Work out the finished part from the listing and answer in its coordinate system (mm). A direction names the side the tool comes from. Round coordinates to 2 decimals unless told otherwise and drop trailing zeros. Order: outer loops, then holes, each group sorted by start corner. A loop starts at its lowest first (then second) coordinate and runs counter-clockwise, first axis right, second up.
from build123d import *

# Parameters (mm, degrees)
FACE_2_R                      = 17
BOSS_EXTRUDE5_DEPTH           = 2
BOSS_EXTRUDE6_START           = -56
BOSS_EXTRUDE6_OUTLINE_R       = 17
BOSS_EXTRUDE6_OUTLINE_R_2     = 10
BOSS_EXTRUDE6_DEPTH           = 54
DRIVER_PIN_BODY_CUT_START     = 9.886859906
DRIVER_PIN_BODY_CUT_OUTLINE_R = 1.5
DRIVER_PIN_BODY_CUT_DEPTH     = 6.113140094
SKETCH5_R                     = 10
SKETCH5_R_2                   = 5
BOSS_EXTRUDE7_DEPTH           = 2
DRIVER_PIN_SKETCH_R           = 1
DRIVER_PIN_SKETCH_R_2         = 0.15
DRIVER_PIN_NECK_EXTRUDE_DEPTH = 1
SKETCH5_6_R                   = 5
SKETCH5_6_R_2                 = 2
CUT_EXTRUDE1_DEPTH            = 1


# Read off the part's stored shape, not the designer's step: Boss-Extrude6, driver_pin_body_cut
with BuildPart() as part:
    # face 2 → Boss-Extrude5 (new body)
    with BuildSketch(Plane.XY):
        Circle(FACE_2_R)
    extrude(amount=-BOSS_EXTRUDE5_DEPTH)

    # Boss-Extrude6 outline → Boss-Extrude6 (add)
    with BuildSketch(Plane.XY.offset(BOSS_EXTRUDE6_START)):
        Circle(BOSS_EXTRUDE6_OUTLINE_R)
        Circle(BOSS_EXTRUDE6_OUTLINE_R_2, mode=Mode.SUBTRACT)
    extrude(amount=BOSS_EXTRUDE6_DEPTH)

    # driver_pin_body_cut outline → driver_pin_body_cut (cut)
    with BuildSketch(Plane(origin=(0, 0, 0), x_dir=(1, 0, 0), z_dir=(0, 1, 0)).offset(DRIVER_PIN_BODY_CUT_START)):
        with Locations((0, 29)):
            Circle(DRIVER_PIN_BODY_CUT_OUTLINE_R)
    extrude(amount=DRIVER_PIN_BODY_CUT_DEPTH, mode=Mode.SUBTRACT)

    # Sketch5 → Boss-Extrude7 (add)
    with BuildSketch(Plane(origin=(0, 0, -56), x_dir=(-1, 0, 0), z_dir=(0, 0, -1))):
        with Locations(Location((0, 0, 0), (0, 0, 180))):
            Circle(SKETCH5_R)
        Circle(SKETCH5_R_2, mode=Mode.SUBTRACT)
    extrude(amount=-BOSS_EXTRUDE7_DEPTH)

    # driver_pin_sketch → driver_pin_neck_extrude (cut)
    # profile 1 of 2: a face of its own
    with BuildSketch(Plane(origin=(0, 17, 0), x_dir=(1, 0, 0), z_dir=(0, 1, 0))):
        with Locations(Location((0, 29, 0), (0, 0, 270))):
            Circle(DRIVER_PIN_SKETCH_R)
        with Locations((0, 29)):
            Circle(DRIVER_PIN_SKETCH_R_2, mode=Mode.SUBTRACT)
    # profile 2 of 2: a face of its own
    with BuildSketch(Plane(origin=(0, 17, 0), x_dir=(1, 0, 0), z_dir=(0, 1, 0))):
        with Locations((0, 29)):
            Circle(DRIVER_PIN_SKETCH_R_2)
    extrude(amount=-DRIVER_PIN_NECK_EXTRUDE_DEPTH, mode=Mode.SUBTRACT)

    # Sketch5<6> → Cut-Extrude1 (cut)
    with BuildSketch(Plane(origin=(0, 0, -56), x_dir=(-1, 0, 0), z_dir=(0, 0, -1))):
        Circle(SKETCH5_6_R)
        with Locations((3.830222216, -3.213938048)):
            Circle(SKETCH5_6_R_2)
        with Locations((-3.830222216, -3.213938048)):
            Circle(SKETCH5_6_R_2)
        with Locations((0, 5)):
            Circle(SKETCH5_6_R_2)
    extrude(amount=-CUT_EXTRUDE1_DEPTH, mode=Mode.SUBTRACT)


solid = part.part
Item 1: Find section C-C (z = -6). Write down the section's boundary in (x, y), plus the area to 3 significant figures.
Item 2: Find section B-B (y = -6). Write down the section's boundary in (x, z), plus the area to 3 significant figures.
Item 3: For a pull along X with two mould halves and no side action, classify faces 1 (the face through (0, 0, 0)), 2 (the face through (-0.383, 16.507, -28.076)), 3 (the face through (9.139, 14.334, -28.392)) as released by +X, released by -X, zero draft, split by the parting line, or undercut.
Item 4: Find section A-A (x = 0). Write down the section's boundary in (y, z).
Item 5: A tool of negligible diameter and unlimited length cuts with its end or side. For faces 4 (the face through (-5.33, -4.54, -55.51)), 5 (the face through (-2.17, -9.76, -28.36)), 6 (the face through (4, 4, -56)), from which of +Z, -Z, +X, -X, +Y, -Y can it reach the whole face along a straight path? Write none if from no direction.
Item 6: Find the intervals of material crossed by line 1 along Z through (x, y) = (1, -5.5); line 2 along X through (y, z) = (-0.5, -12); line 3 along Y through (x, z) = (0, -22.5), in increasing order.
Item 7: Find section D-D (y = 0). Write down the section's boundary in (x, z).
Item 8: Given pin 1 (1.5 mm diameter, centred on y = -12, z = -36.5, fed in from +X); pin 2 (1 mm diameter, centred on x = -13.5, y = 12, fed in from +Z); pin 3 (5 mm diameter, centred on x = 9.5, z = -48, fed in from +Y); pin 4 (8 mm diameter, centred on y = 13, z = -21.5, fed in from +X), each flat-ended and moving along its own axis, determine where each tip first touches the part or whether it passes through.
Model answer:
1. outline: circle Ø34 at (0, 0); hole circle Ø20 at (0, 0)
1. area: 594 mm2
2. outline: (-15.91, -56) - (15.91, -56) - (15.91, 0) - (-15.91, 0) - close; hole (-8, -54) - (8, -54) - (8, -2) - (-8, -2) - close
2. area: 949 mm2
3. face 1: zero draft
3. face 2: undercut
3. face 3: split by the parting line
4. outline: (-17, -56) - (-5, -56) - (-5, -54) - (-10, -54) - (-10, -2) - (10, -2) - (10, -27.5) - (16, -27.5) - (16, -28) - (17, -28) - (17, 0) - (-17, 0) - close; (5, -55) - (7, -55) - (7, -56) - (17, -56) - (17, -30) - (16, -30) - (16, -30.5) - (10, -30.5) - (10, -54) - (5, -54) - close
5. face 4: -Z
5. face 5: none
5. face 6: -Z, +X, -X, +Y, -Y
6. line 1: z = -56 to -54, -2 to 0
6. line 2: x = -16.99 to -9.99, 9.99 to 16.99
6. line 3: y = -17 to -10, 10 to 17
7. outline: (-17, -56) - (-5, -56) - (-5, -54) - (-10, -54) - (-10, -2) - (10, -2) - (10, -54) - (5, -54) - (5, -56) - (17, -56) - (17, 0) - (-17, 0) - close
8. pin 1: stops at x = 12.75
8. pin 2: passes through
8. pin 3: stops at y = 15.49
8. pin 4: stops at x = 14.42
